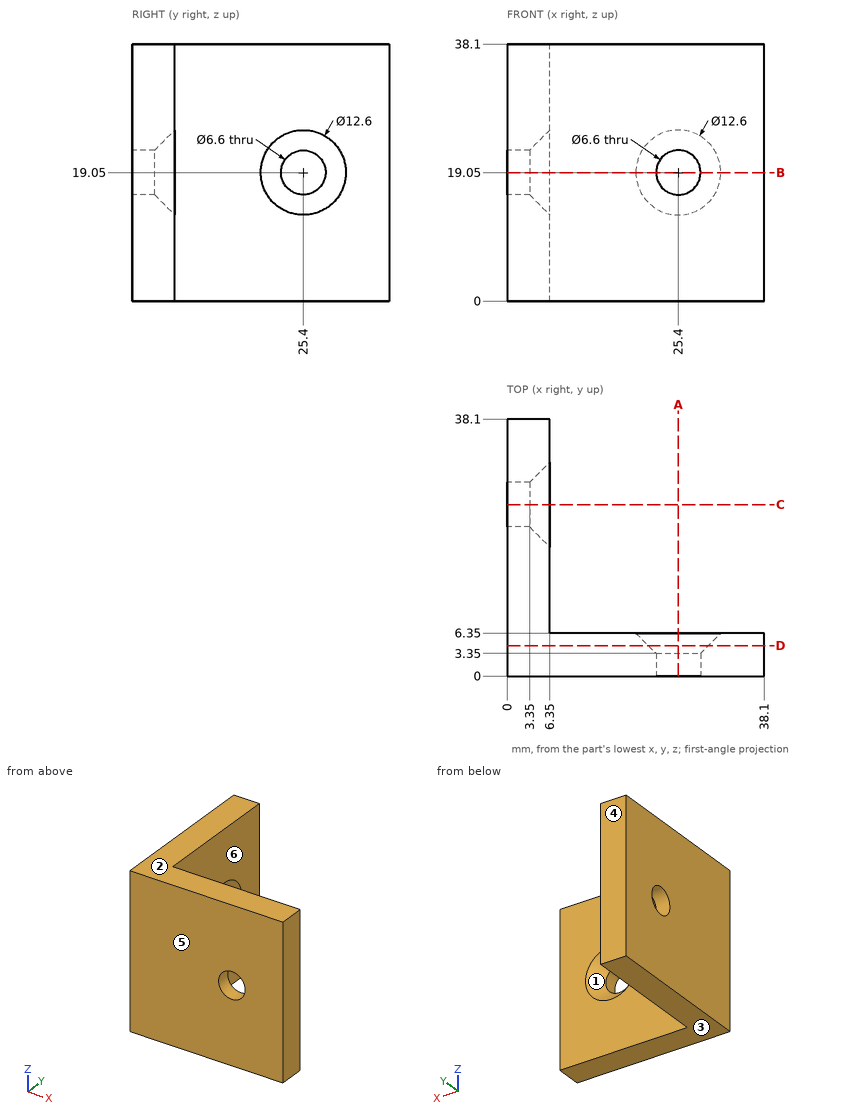
Geometry: see drawing. Coordinates: mm, zero at the bounding-box minimum. A direction names the side the tool comes from. Round coordinates to 2 decimals unless told otherwise and drop trailing zeros. Loops run counter-clockwise (first coordinate to the right, second up) from the corner with the lowest first, then second, coordinate; pieces in that order, holes last.
(1) Pull-direction query (Z, two-part tool) for the marked faces 1, 2, 3 and 4; classes: +Z half, -Z half, draft (parallel to the pull), parting line (faces both ways), or undercut.
From the geometry:
face 1: undercut
face 2: +Z half
face 3: -Z half
face 4: draft
(2) Material intervals for probe 1 along X at (y, z) = (2.45, 19.05); probe 2 along Y at (x, z) = (15.5, 9), sorted ascending.
From the geometry:
probe 1: x = 0 to 22.1, 28.7 to 38.1
probe 2: y = 0 to 6.35
(3) Section query D-D (y = 4.5). Output: boundary loops of the cut face in (x, z), and give its area (3 significant figures).
From the geometry:
outline: (0, 0) - (38.1, 0) - (38.1, 38.1) - (0, 38.1) - close; hole circle Ø8.9 at (25.4, 19.05)
area: 1,390 mm2
(4) Section query B-B (z = 19.05). Output: boundary loops of the cut face in (x, y).
From the geometry:
outline: (0, 0) - (22.1, 0) - (22.1, 3.35) - (19.1, 6.35) - (6.35, 6.35) - (6.35, 19.1) - (3.35, 22.1) - (0, 22.1) - close; (0, 28.7) - (3.35, 28.7) - (6.35, 31.7) - (6.35, 38.1) - (0, 38.1) - close; (28.7, 0) - (38.1, 0) - (38.1, 6.35) - (31.7, 6.35) - (28.7, 3.35) - close
(5) Contact query for flat-ended pins moving along their axis: pin 1 Ø16 at (x, z) = (20.5, 28) entering from +Y; pin 2 Ø7.5 at (x, z) = (25.4, 19.05) entering from -Y; pin 3 Ø1.5 at (x, z) = (26, 14) entering from +Y; pin 4 Ø8 at (y, z) = (16.5, 15) entering from +X. Output: stop coordinate, or through.
From the geometry:
pin 1: stops at y = 6.35
pin 2: stops at y = 0
pin 3: stops at y = 5.89
pin 4: stops at x = 6.35
(6) Access query for the marked faces 5 and 6. Directions: +Z, -Z, +X, -X, +Y, -Y. A direction counts if a zero-diameter tool reaches every point of the face in a straight line with its end or side. Return the directions, or none.
From the geometry:
face 5: +Z, -Z, +X, -X, -Y
face 6: +Z, -Z, +X, +Y
(7) Section query A-A (x = 25.4). Output: boundary loops of the cut face in (y, z), and give its area (3 significant figures).
From the geometry:
outline: (0, 0) - (6.35, 0) - (6.35, 12.75) - (3.35, 15.75) - (0, 15.75) - close; (0, 22.35) - (3.35, 22.35) - (6.35, 25.35) - (6.35, 38.1) - (0, 38.1) - close
area: 191 mm2
